The listing builds one solid part. Answer for the finished solid, in the listing's coordinates (mm). Round coordinates to 2 decimals unless told otherwise and drop trailing zeros. Order: outer loops, then holes, each group sorted by start corner. A loop starts at its lowest first (then second) coordinate and runs counter-clockwise, first axis right, second up. Notation, with made-up numbers: M 58.5,37.25 L 82.5,37.25 A9 ccw 82.5,42.25 Z; hole C 32.5,11.25 d11. An arc over 180 degrees is marked long. Put each result on its own line as item: value. Start each with the question number.
1. The part is cut by section D-D (z = -62.5). Give the vertices of the cut face in (x, y) (3 decimals).
2. Each of these flat-tipped pins is pushed along its axis until it touches: pin 1 Ø1.6 at (y, z) = (1, 61.5) entering from +X; pin 2 Ø0.6 at (y, z) = (2, 55.5) entering from +X; pin 3 Ø1 at (y, z) = (1, -43) entering from +X. Where does it stop, or does it pass through?
3. The part is cut by section A-A (x = 0). Give the vertices of the cut face in (y, z) (3 decimals).
4. The part is cut by section C-C (y = 2.1). Count the separate pieces of the cut face and the enclosed holes in it, then the cut area to 3 significant figures.
5. The part is cut by section B-B (z = 32). Give the vertices of the cut face in (x, y) (3 decimals), then the cut area to 3 significant figures.
6. The mould has two halves that part along Z. Classify faces 1 (the face through (-57.519, 1.61, 38.347)), 2 (the face through (-1.9, 1.61, 58.12)), 3 (the face through (-84.323, 1.565, -10.709)), 4 (the face through (-1, 0, -11)): +Z half, -Z half, draft (parallel to the pull), parting line (faces both ways), or undercut.
7. Consider line 1 (X direction, y = 2.8, z = -75.5); line 2 (X direction, y = 2.7, z = -43); line 3 (X direction, y = 1.35, z = 50) (3 decimals). Determine where each line is inside the solid, lowest interval first.
from build123d import *

# Parameters (mm, degrees)
BOSS_EXTRUDE4_DEPTH  = 3.175
SKETCH17_R           = 8.5
BOSS_EXTRUDE5_DEPTH  = 3.175
M3_CLEARANCE_HOLE3_D = 3
M3_CLEARANCE_HOLE1_D = 3.1
M3_CLEARANCE_HOLE4_D = 2.95
M3_CLEARANCE_HOLE2_D = 3.1
CUT_EXTRUDE1_DEPTH   = 121.250075364
BOSS_EXTRUDE6_DEPTH  = 3.175
FILLET1_R            = 2
FILLET3_R            = 1
SKETCH23_R           = 4.95
CUT_EXTRUDE2_DEPTH   = 121.250075364


with BuildPart() as part:
    # Sketch1 → Boss-Extrude4 (new body)
    with BuildSketch(Plane(origin=(0, 0, 0), x_dir=(1, 0, 0), z_dir=(0, 1, 0))):
        with BuildLine():
            Line((-62.799553621, 32.496136604), (-73.969425011, 32.691107434))
            Line((-73.969425011, 32.691107434), (-77.053684287, 35.88495141))
            ThreePointArc((-77.053684287, 35.88495141), (-84.36642289, 10.358894189), (-83.446216027, -16.178041625))
            Line((-83.446216027, -16.178041625), (-79.680911643, -13.825218315))
            Line((-79.680911643, -13.825218315), (-69.484649137, -16.179210996))
            Line((-69.484649137, -16.179210996), (-43.094490772, -58.412292655))
            Line((-43.094490772, -58.412292655), (-43.094490772, -64.826600275))
            Line((-43.094490772, -64.826600275), (-34, -64.826600275))
            Line((-34, -64.826600275), (-34, -58.55))
            Line((-34, -58.55), (-34, -53.55))
            Line((-34, -53.55), (-28, -53.55))
            Line((-28, -53.55), (-28, -58.55))
            Line((-28, -58.55), (28, -58.55))
            Line((28, -58.55), (28, -53.55))
            Line((28, -53.55), (34, -53.55))
            Line((34, -53.55), (34, -58.55))
            Line((34, -58.55), (34, -64.826600275))
            Line((34, -64.826600275), (43.094490772, -64.826600275))
            Line((43.094490772, -64.826600275), (43.094490772, -58.412292655))
            Line((43.094490772, -58.412292655), (69.484649137, -16.179210996))
            Line((69.484649137, -16.179210996), (79.680911643, -13.825218315))
            Line((79.680911643, -13.825218315), (83.446216027, -16.178041625))
            ThreePointArc((83.446216027, -16.178041625), (84.610662337, -8.126242604), (85, 0))
            ThreePointArc((85, 0), (82.98964744, 18.377116688), (77.053684287, 35.88495141))
            Line((77.053684287, 35.88495141), (73.969425011, 32.691107434))
            Line((73.969425011, 32.691107434), (62.799553621, 32.496136604))
            Line((62.799553621, 32.496136604), (30.284668021, 63.895396642))
            Line((30.284668021, 63.895396642), (30.089697191, 75.065268032))
            Line((30.089697191, 75.065268032), (33.173956467, 78.259112008))
            ThreePointArc((33.173956467, 78.259112008), (0, 85), (-33.173956467, 78.259112008))
            Line((-33.173956467, 78.259112008), (-30.089697191, 75.065268032))
            Line((-30.089697191, 75.065268032), (-30.284668021, 63.895396642))
            Line((-30.284668021, 63.895396642), (-62.799553621, 32.496136604))
        make_face()
    extrude(amount=BOSS_EXTRUDE4_DEPTH)

    # Sketch17 → Boss-Extrude5 (add)
    with BuildSketch(Plane(origin=(0, 3.175, 0), x_dir=(1, 0, 0), z_dir=(0, 1, 0))):
        with Locations((0, -53.55)):
            Circle(SKETCH17_R)
    extrude(amount=-BOSS_EXTRUDE5_DEPTH)

    # M3 Clearance Hole3 (through all)
    with Locations(Plane(origin=(0, 0, 0), x_dir=(-1, 0, 0), z_dir=(0, -1, 0))):
        with Locations((36.415, -50), (36.415, -38), (-36.415, -50), (-36.415, -38)):
            Hole(M3_CLEARANCE_HOLE3_D / 2)

    # M3 Clearance Hole1 (through all)
    with Locations(Plane(origin=(0, 3.175, 0), x_dir=(1, 0, 0), z_dir=(0, 1, 0))):
        with Locations((-78.542321426, -8.49139241), (78.542321426, -8.49139241), (74.155025063, 27.240269049), (-74.155025063, 27.240269049)):
            Hole(M3_CLEARANCE_HOLE1_D / 2)

    # M3 Clearance Hole4 (through all)
    with Locations(Plane(origin=(0, 0, 0), x_dir=(-1, 0, 0), z_dir=(0, -1, 0))):
        with Locations((-67.099301622, -15.278865202), (-50.141885166, -42.416404279), (-61.062544382, 30.698137949), (-38.043670771, 52.927205804), (50.141885166, -42.416404279), (67.099301622, -15.278865202), (38.043670771, 52.927205804), (61.062544382, 30.698137949)):
            Hole(M3_CLEARANCE_HOLE4_D / 2)

    # M3 Clearance Hole2 (through all)
    with Locations(Plane(origin=(0, 3.175, 0), x_dir=(1, 0, 0), z_dir=(0, 1, 0))):
        with Locations((27, 76.497766718), (-27, 76.497766718)):
            Hole(M3_CLEARANCE_HOLE2_D / 2)

    # Sketch20 → Cut-Extrude1 (cut, through all)
    with BuildSketch(Plane(origin=(0, 3.175, 0), x_dir=(1, 0, 0), z_dir=(0, 1, 0))):
        with BuildLine():
            Line((-14.64850035, 45.5), (-14.64850035, 40.5))
            ThreePointArc((-14.64850035, 40.5), (-16.14850035, 39), (-17.64850035, 40.5))
            Line((-17.64850035, 40.5), (-17.64850035, 45.5))
            ThreePointArc((-17.64850035, 45.5), (-16.14850035, 47), (-14.64850035, 45.5))
        make_face()
        with BuildLine():
            Line((14.64850035, 45.5), (14.64850035, 40.5))
            ThreePointArc((14.64850035, 40.5), (16.14850035, 39), (17.64850035, 40.5))
            Line((17.64850035, 40.5), (17.64850035, 45.5))
            ThreePointArc((17.64850035, 45.5), (16.14850035, 47), (14.64850035, 45.5))
        make_face()
    extrude(amount=-CUT_EXTRUDE1_DEPTH, mode=Mode.SUBTRACT)

    # Sketch22 → Boss-Extrude6 (add)
    with BuildSketch(Plane(origin=(0, 3.175, 0), x_dir=(1, 0, 0), z_dir=(0, 1, 0))):
        Polygon((-30.284668021, 63.895396642), (-30.245177733, 66.157793715), (-65.061950694, 32.535626892), (-62.799553621, 32.496136604), align=None)
        Polygon((-69.484649137, -16.179210996), (-71.689396914, -15.670204865), (-43.094490772, -61.431620518), (-43.094490772, -58.412292655), align=None)
        Polygon((43.094490772, -61.431620518), (71.689396914, -15.670204865), (69.484649137, -16.179210996), (43.094490772, -58.412292655), align=None)
        Polygon((65.061950694, 32.535626892), (30.245177733, 66.157793715), (30.284668021, 63.895396642), (62.799553621, 32.496136604), align=None)
    extrude(amount=-BOSS_EXTRUDE6_DEPTH)

    # Fillet1
    fillet1_edges = [part.edges().sort_by_distance(p)[0] for p in [
        (-30.245177733, 1.5875, -66.157793715),
        (-65.061950694, 1.5875, -32.535626892),
        (-71.689396914, 1.5875, 15.670204865),
        (-43.094490772, 1.5875, 61.431620518),
        (43.094490772, 1.5875, 61.431620518),
        (71.689396914, 1.5875, 15.670204865),
        (65.061950694, 1.5875, -32.535626892),
        (30.245177733, 1.5875, -66.157793715),
        (30.089697191, 1.5875, -75.065268032),
        (73.969425011, 1.5875, -32.691107434),
        (79.680911643, 1.5875, 13.825218315),
        (28, 1.5875, 58.55),
        (-28, 1.5875, 58.55),
        (-79.680911643, 1.5875, 13.825218315),
        (-73.969425011, 1.5875, -32.691107434),
        (-30.089697191, 1.5875, -75.065268032),
    ]]
    fillet(fillet1_edges, radius=FILLET1_R)

    # Fillet3
    fillet3_edges = [part.edges().sort_by_distance(p)[0] for p in [
        (33.173956467, 1.5875, -78.259112008),
        (77.053684287, 1.5875, -35.88495141),
        (83.446216027, 1.5875, 16.178041625),
        (43.094490772, 1.5875, 64.826600275),
        (34, 1.5875, 64.826600275),
        (34, 1.5875, 53.55),
        (28, 1.5875, 53.55),
        (-28, 1.5875, 53.55),
        (-34, 1.5875, 53.55),
        (-34, 1.5875, 64.826600275),
        (-43.094490772, 1.5875, 64.826600275),
        (-83.446216027, 1.5875, 16.178041625),
        (-77.053684287, 1.5875, -35.88495141),
        (-33.173956467, 1.5875, -78.259112008),
        (-6.873863542, 1.5875, 58.55),
        (6.873863542, 1.5875, 58.55),
    ]]
    fillet(fillet3_edges, radius=FILLET3_R)

    # Sketch23 → Cut-Extrude2 (cut, through all)
    with BuildSketch(Plane(origin=(0, 3.175, 0), x_dir=(1, 0, 0), z_dir=(0, 1, 0))):
        with Locations(Location((0, -53.55, 0), (0, 0, 270))):
            Circle(SKETCH23_R)
    extrude(amount=-CUT_EXTRUDE2_DEPTH, mode=Mode.SUBTRACT)


solid = part.part
Resolved:
1. outline: M -34.033,0 L 34.033,0 L 34.033,3.175 L -34.033,3.175 Z
2. pin 1: x = 43.55
2. pin 2: x = 46.99
2. pin 3: x = 54.74
3. outline: M 0,-85 L 3.175,-85 L 3.175,48.6 L 0,48.6 Z; M 0,58.5 L 3.175,58.5 L 3.175,62.05 L 0,62.05 Z
4. separate pieces: 1
4. enclosed holes: 21
4. area: 17,100 mm2
5. outline: M -61.485,0 L 61.485,0 L 61.485,3.175 L -61.485,3.175 Z
5. area: 390 mm2
6. face 1: +Z half
6. face 2: undercut
6. face 3: parting line
6. face 4: draft
7. line 1: -30.53 to -28.19, -25.81 to 25.81, 28.19 to 30.53
7. line 2: -54.23 to -17.65, -14.65 to 14.65, 17.65 to 54.23
7. line 3: -50.238 to -37.915, -34.915 to -3.45, 3.45 to 34.915, 37.915 to 50.238
